Autodesk Inventor part; units mm, degrees
ref_plane "YZ Plane" through (0, 0, 0) normal (1, 0, 0) x (0, 1, 0)
ref_plane "XZ Plane" through (0, 0, 0) normal (0, 1, 0) x (-1, 0, 0)
ref_plane "XY Plane" through (0, 0, 0) normal (0, 0, 1) x (1, 0, 0)
sketch "Sketch1" plane through (0, 0, 0) normal (0, 0, 1) x (1, 0, 0)
  line L0 (1604.4809, 6805.3292) -> (1804.4809, 6805.3292)
  line L1 (1804.4809, 6805.3292) -> (1804.4809, 6605.3292)
  line L2 (1804.4809, 6605.3292) -> (1604.4809, 6605.3292)
  line L3 (1604.4809, 6605.3292) -> (1604.4809, 6805.3292)
  point P0 (0, 0)
  dimension "d0" = 200
  dimension "d1" = 200
extrude "Extrusion1" add sketch "Sketch1" along normal blind 200
sketch "Sketch2" plane through (0, 0, 200) normal (0, 0, 1) x (1, 0, 0)
  line L0 (1804.4809, 6805.3292) -> (1604.4809, 6805.3292)
  line L1 (1604.4809, 6605.3292) -> (1804.4809, 6605.3292)
  circle A0 centre (1704.4809, 6705.3292) radius 45
  point P0 (0, 0)
  dimension "d4" = 90
extrude "Extrusion2" add sketch "Sketch2" along normal blind 1100
sketch "Sketch4" plane through (1804.4809, 6605.3292, 0) normal (1, 0, 0) x (0, 0, -1)
  line L0 (0, 200) -> (-200, 200)
  line L1 (-100, 200) -> (-100, 0)
  line L2 (0, 0) -> (-200, 0)
  circle A0 centre (-100, 100) radius 45
  point P0 (0, -6605.3292)
  dimension "d12" = 90
extrude "Extrusion4" cut sketch "Sketch4" against normal blind 200
mirror "Mirror1" about plane through (1704.4809, 6705.3292, 1300) normal (0, 0, 1) of "Extrusion2", "Extrusion1", "Extrusion4"
thread "Thread1"
properties part number "srodek"
For this review, take the finished solid that the model builds, in its own axes (mm). A direction names the side the tool comes from. Give positions to 0.01 mm unless a question says otherwise; leave off trailing zeros. Loops run counter-clockwise (first coordinate to the right, second up) from the corner with the lowest first, then second, coordinate; pieces in that order, holes last. Notation, with made-up numbers: M 77,34.25 L 131,34.25 A21 ccw 131,50.25 Z; hole C 32,87.5 d9. An arc over 180 degrees is marked long. One line per item, written item: value. Start each with the question number.
Q1. Add section D-D (z = 2208). Give the boundary of the cut face in (x, y), and give its area (3 significant figures).
Q2. Add section A-A (y = 6637.5). Give the boundary of the cut face in (x, z).
Q3. Add section C-C (x = 1701). Give the boundary of the cut face in (y, z), and give its area (3 significant figures).
Q4. For L1, parallel to Z at x = 1790.5, y = 6700.5; L2, parallel to Z at x = 1770.5, y = 6702; L3, parallel to Y at x = 1675, z = 2500, list the stretches that pass through material, from the lowest coordinate up.
Q5. Machinability: for faces 4 (the face through (1706, 6605.329, 99)), 5 (the face through (1668.77, 6732.71, 1284.6)), which of the approach directions +Z, -Z, +X, -X, +Y, -Y give a long, thin tool a straight path to every point of the face, cutting with its end or side? Answer none if there is none.
Q6. Draft analysis for pull direction Z (two halves, no side actions). For faces 1 (the face through (1703, 6707, 0)), 2 (the face through (1804.481, 6707, 54)), 3 (the face through (1705.88, 6732.71, 2464.29)), state which applies: released by +Z, released by -Z, zero draft, split by the parting line, or undercut.
Q7. Clearance check with flat-ended pins moving along their axes: pin 1 Ø1.5 at (x, z) = (1730.5, 1958) entering from +Y; pin 2 Ø6 at (y, z) = (6748.5, 2250.5) entering from +X; pin 3 Ø4 at (y, z) = (6734.5, 517.5) entering from +X. State where each tip first meets the part, or that it passes through.
Q8. Add section B-B (z = 100). Give the boundary of the cut face in (x, y).
Reply:
1. outline: C 1704.48,6705.33 d90
1. area: 6,360 mm²
2. outline: M 1604.48,0 L 1804.48,0 L 1804.48,200 L 1604.48,200 Z; M 1604.48,2400 L 1804.48,2400 L 1804.48,2600 L 1604.48,2600 Z
3. outline: M 6605.33,0 L 6805.33,0 L 6805.33,200 L 6750.19,200 L 6750.19,2400 L 6805.33,2400 L 6805.33,2600 L 6605.33,2600 L 6605.33,2400 L 6660.46,2400 L 6660.46,200 L 6605.33,200 Z; hole C 6705.33,100 d90; hole C 6705.33,2500 d90
3. area: 265,000 mm²
4. L1: 0 to 55.26, 144.74 to 200, 2400 to 2455.26, 2544.74 to 2600
4. L2: 0 to 55.12, 144.88 to 200, 2400 to 2455.12, 2544.88 to 2600
4. L3: 6605.33 to 6660.33, 6750.33 to 6805.33
5. face 4: +Z, -Z, +X, -X, -Y
5. face 5: none
6. face 1: released by -Z
6. face 2: zero draft
6. face 3: undercut
7. pin 1: y = 6742.56
7. pin 2: x = 1724.76
7. pin 3: x = 1740.35
8. outline: M 1604.48,6605.33 L 1804.48,6605.33 L 1804.48,6660.33 L 1604.48,6660.33 Z; M 1604.48,6750.33 L 1804.48,6750.33 L 1804.48,6805.33 L 1604.48,6805.33 Z
